Study the drawing (mm; zero at the part's minimum x, y, z) and answer. A direction names the side the tool comes from. Coordinates: 2 decimals unless noted, no trailing zeros. Write each loop counter-clockwise with the first axis right and the second up, starting at its lowest first coordinate (ties: lowest second). Pieces come first, ordered by that corner, then holes. Notation, with made-up numbers: (82.5, -12.5) -> (90.5, -12.5) arc R18 cw to (90.5, 1.5) -> close; hole circle Ø2 at (66, 35). An arc over 180 degrees is marked (long way). Write item = value, one per line. Start each with the question number.
1) Flat-ended cylindrical pins translate along their axes: pin 1 Ø5 at (y, z) = (6.5, 29) entering from -X; pin 2 Ø10 at (x, z) = (13, 19.5) entering from -Y; pin 3 Ø1 at (x, z) = (12.5, 18.5) entering from +Y. Find the tip coordinate at first contact, or state that the pin passes through.
2) A tool of negligible diameter and unlimited length cuts with its end or side. For the marked faces 1 and 2, from which of +Z, -Z, +X, -X, +Y, -Y can it reach the whole face along a straight path? Write none if from no direction.
3) Section A-A (y = 6) is taken. Determine the outline of the cut face in (x, z).
4) Find the intervals of material crossed by line 1 along X through (y, z) = (1, 28.5); line 2 along Y through (x, z) = (16, 1.2); line 3 along Z through (x, y) = (4, 1.35), in increasing order. Write a range as from..to.
5) Section B-B (x = 4) is taken. Determine the outline of the cut face in (y, z).
6) Section D-D (y = 2.5) is taken. Determine the outline of the cut face in (x, z).
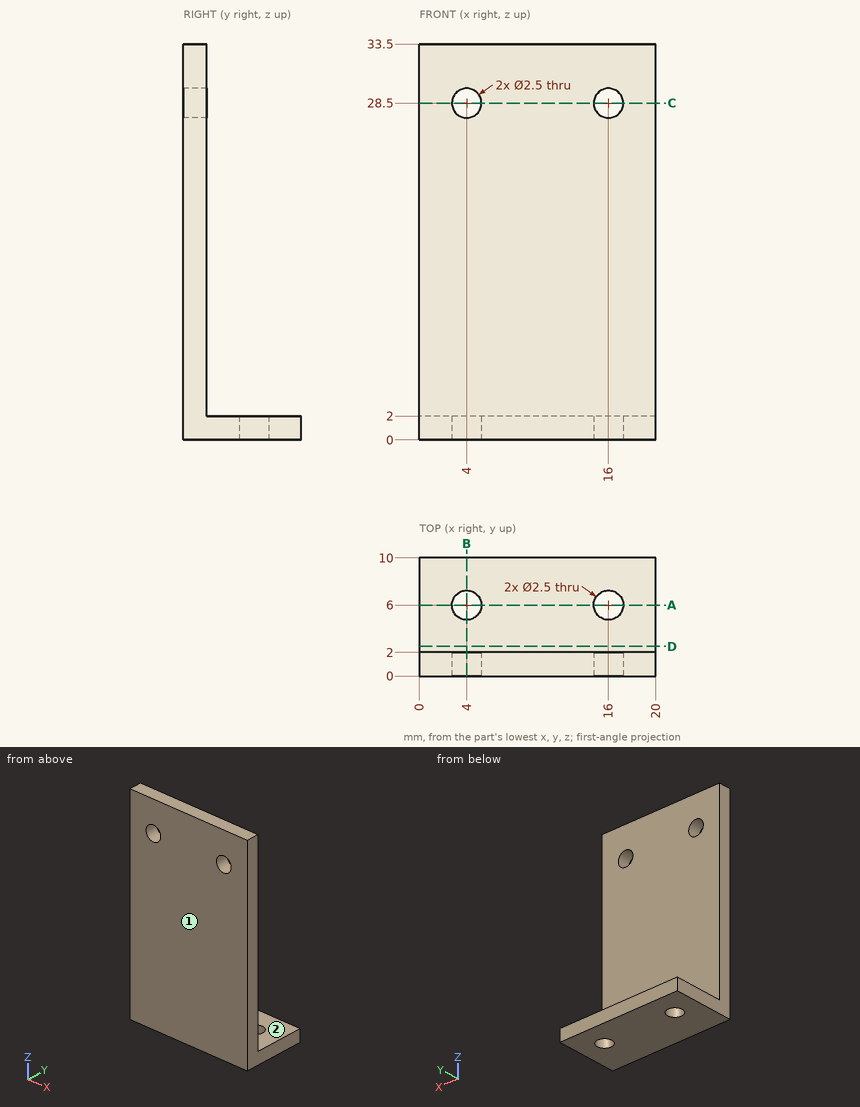
Answer key:
q1.pin_1 = through
q1.pin_2 = 0
q1.pin_3 = 2
q2.face_1 = +Z, -Z, +X, -X, -Y
q2.face_2 = +Z, +X, -X, +Y
q3.outline = (0, 0) -> (2.75, 0) -> (2.75, 2) -> (0, 2) -> close; (5.25, 0) -> (14.75, 0) -> (14.75, 2) -> (5.25, 2) -> close; (17.25, 0) -> (20, 0) -> (20, 2) -> (17.25, 2) -> close
q4.line_1 = 0..2.75, 5.25..14.75, 17.25..20
q4.line_2 = 0..4.75, 7.25..10
q4.line_3 = 0..27.25, 29.75..33.5
q5.outline = (0, 0) -> (4.75, 0) -> (4.75, 2) -> (2, 2) -> (2, 27.25) -> (0, 27.25) -> close; (0, 29.75) -> (2, 29.75) -> (2, 33.5) -> (0, 33.5) -> close; (7.25, 0) -> (10, 0) -> (10, 2) -> (7.25, 2) -> close
q6.outline = (0, 0) -> (20, 0) -> (20, 2) -> (0, 2) -> close
